```python
from build123d import *

# Parameters (mm, degrees)
SKETCH2_R           = 8
BASE_EXTRUDE_DEPTH  = 19.05
SKETCH3_R           = 2.5
BOSS_EXTRUDE1_DEPTH = 2.54
SKETCH5_R           = 1.5
BOSS_EXTRUDE2_DEPTH = 8
CUT_EXTRUDE1_START  = -8
CUT_EXTRUDE1_DEPTH  = 8
SKETCH7_R           = 7
BOSS_EXTRUDE3_DEPTH = 23.25
BOSS_EXTRUDE4_DEPTH = 2


with BuildPart() as part:
    # Sketch2 → Base-Extrude (new body)
    with BuildSketch(Plane.XY):
        Circle(SKETCH2_R)
    extrude(amount=-BASE_EXTRUDE_DEPTH)

    # Sketch3 → Boss-Extrude1 (add)
    with BuildSketch(Plane.XY):
        Circle(SKETCH3_R)
    extrude(amount=BOSS_EXTRUDE1_DEPTH)

    # Sketch5 → Boss-Extrude2 (add)
    with BuildSketch(Plane.XY.offset(2.54)):
        Circle(SKETCH5_R)
    extrude(amount=BOSS_EXTRUDE2_DEPTH)

    # Sketch6 → Cut-Extrude1 (cut)
    with BuildSketch(Plane.XY.offset(10.54).offset(CUT_EXTRUDE1_START)):
        with BuildLine():
            Line((-2.334314707, 0.894971982), (2.334314707, 0.894971982))
            ThreePointArc((2.334314707, 0.894971982), (0, 2.5), (-2.334314707, 0.894971982))
        make_face()
    extrude(amount=CUT_EXTRUDE1_DEPTH, mode=Mode.SUBTRACT)

    # Sketch7 → Boss-Extrude3 (add)
    with BuildSketch(Plane(origin=(0, 0, -19.05), x_dir=(-1, 0, 0), z_dir=(0, 0, -1))):
        with Locations(Location((0, 0, 0), (0, 0, 180))):
            Circle(SKETCH7_R)
    extrude(amount=BOSS_EXTRUDE3_DEPTH)

    # Sketch8 → Boss-Extrude4 (add)
    with BuildSketch(Plane(origin=(0, 0, -42.3), x_dir=(-1, 0, 0), z_dir=(0, 0, -1))):
        with BuildLine():
            Line((3.2, 2.704829015), (3.2, -2.704829015))
            ThreePointArc((3.2, -2.704829015), (-4.19, 0), (3.2, 2.704829015))
        make_face()
    extrude(amount=BOSS_EXTRUDE4_DEPTH)


solid = part.part
```
Here's how the part is built. I have some questions about the finished solid (model axes, mm). A direction names the side the tool comes from. Round coordinates to 2 decimals unless told otherwise and drop trailing zeros. Write each loop counter-clockwise with the first axis right and the second up, starting at its lowest first coordinate (ties: lowest second). Pieces come first, ordered by that corner, then holes. Notation, with made-up numbers: M 28.5,-15 L 71.5,-15 A16 cw 71.5,-10 Z; hole C 33.5,-23.5 d8. An arc over 180 degrees is marked long. Answer as CSV lines item,"result". Start each with the question number.
1. Suppose I cut it at D-D on y = -5.25. Write out the boundary of the cut face in (x, z), then the cut area to 3 significant figures.
2. I need wall thicknesses on probe 1 along Z at (x, y) = (4.75, 5.25); probe 2 along Z at (x, y) = (-2, -2.5); probe 3 along X at (y, z) = (-4.25, -27). Which ranges of each line are inside material? Lowest first, please.
3. Suppose I cut it at C-C on z = -8.5. Write out the boundary of the cut face in (x, y), then the cut area to 3 significant figures.
4. Suppose I cut it at B-B on x = 0. Write out the boundary of the cut face in (y, z), then the cut area to 3 significant figures.
5. I'm going to push flat-ended pins straight in: pin 1 Ø4 at (x, z) = (4, 1) entering from -Y; pin 2 Ø3 at (y, z) = (3, -5) entering from -X; pin 3 Ø2.5 at (x, z) = (0, 8) entering from +Y (3 decimals). Where does each tip first touch, or does it pass through?
6. On a 3-axis mill with a long thin cutter (end or side, diameter ignored), from which of +Z, -Z, +X, -X, +Y, -Y can I reach the whole of each face in a straight line? I mean faces 1 (the flat face through (0, 0.895, 6)), 2 (the cylindrical face through (4.188, -0.143, -43.286)), 3 (the flat face through (-3.2, 0, -43)). Say none if no direction works.
7. Suppose I cut it at A-A on y = 0. Write out the boundary of the cut face in (x, z).
Check result:
1,outline,"M -6.04,-19.05 L -4.63,-19.05 L -4.63,-42.3 L 4.63,-42.3 L 4.63,-19.05 L 6.04,-19.05 L 6.04,0 L -6.04,0 Z"
1,area,"445 mm2"
2,probe 1,"z = -19.05 to 0"
2,probe 2,"z = -44.3 to 0"
2,probe 3,"x = -5.56 to 5.56"
3,outline,"C 0,0 d16"
3,area,"201 mm2"
4,outline,"M -8,-19.05 L -7,-19.05 L -7,-42.3 L -4.19,-42.3 L -4.19,-44.3 L 4.19,-44.3 L 4.19,-42.3 L 7,-42.3 L 7,-19.05 L 8,-19.05 L 8,0 L 2.5,0 L 2.5,2.54 L 0.89,2.54 L 0.89,10.54 L -1.5,10.54 L -1.5,2.54 L -2.5,2.54 L -2.5,0 L -8,0 Z"
4,area,"679 mm2"
5,pin 1,"stops at y = -7.67"
5,pin 2,"stops at x = -7.86"
5,pin 3,"stops at y = 0.895"
6,face 1,"+Z, +X, -X, +Y"
6,face 2,"-Z"
6,face 3,"-Z, -X, +Y, -Y"
7,outline,"M -8,-19.05 L -7,-19.05 L -7,-42.3 L -3.2,-42.3 L -3.2,-44.3 L 4.19,-44.3 L 4.19,-42.3 L 7,-42.3 L 7,-19.05 L 8,-19.05 L 8,0 L 2.5,0 L 2.5,2.54 L 1.5,2.54 L 1.5,10.54 L -1.5,10.54 L -1.5,2.54 L -2.5,2.54 L -2.5,0 L -8,0 Z"
